The model under review builds one solid part; all positions refer to its coordinate system, in mm. Round coordinates to 2 decimals unless told otherwise and drop trailing zeros. Loops run counter-clockwise (first coordinate to the right, second up) from the corner with the lowest first, then second, coordinate; pieces in that order, holes last. Notation, with made-up numbers: M -31.75,67 L 5.25,67 A34 ccw 5.25,99 Z; hole C 52.25,64 d6. An arc over 180 degrees is marked long. Answer as a JSON object with one key per item and string values. Group by question number.
Item 1: Consider section B-B (x = 0). Give the boundary of the cut face in (y, z), and give its area (3 significant figures).
Item 2: Consider section D-D (x = 24). Give the boundary of the cut face in (y, z), and give its area (3 significant figures).
Item 3: Insertion check: P1, Ø1.8, axis at x = 33, z = -31, coming from the -Y side; P2, Ø1.6, axis at x = 38, y = 2, coming from the +Z side; P3, Ø0.9, axis at y = 2, z = -27, coming from the -X side; P4, Ø1.6, axis at x = -38.5, y = 2, coming from the -Z side. Each pin has a flat end and moves straight along its axis. Give the tip position at first contact, or say it passes through.
Item 4: Consider section C-C (z = 6.5). Give the boundary of the cut face in (x, y), and give its area (3 significant figures).
Item 5: Consider section A-A (z = 29). Give the boundary of the cut face in (x, y), and give its area (3 significant figures).
Item 6: To check wall thickness, follow line 1 (Z direction, x = 16.5, y = 1.85); line 2 (Z direction, x = 4, y = 1.3); line 3 (Z direction, x = -15.5, y = 0.75). State the ranges of each line that lie inside material, in increasing order.
```python
from build123d import *

# Parameters (mm, degrees)
SKETCH_2_R          = 11.05
SKETCH_2_R_2        = 2
SKETCH_2_R_3        = 4.5
SKETCH_2_R_4        = 1.5
EXTRUDE_1_DEPTH     = 3
SKETCH_3_R          = 1
CUT_EXTRUDE_1_DEPTH = 54.235326617
FILLET_1_R          = 1
FILLET_2_R          = 2


with BuildPart() as part:
    # 草图2 → 凸台-拉伸1 (new body)
    with BuildSketch(Plane(origin=(0, 0, 0), x_dir=(1, 0, 0), z_dir=(0, 1, 0))):
        Polygon((-37, 35), (37, 35), (37, 22.5), (40, 22.5), (40, 7.5), (37, 7.5), (37, -7.5), (40, -7.5), (40, -22.5), (37, -22.5), (37, -35), (-37, -35), (-37, -22.5), (-40, -22.5), (-40, -7.5), (-37, -7.5), (-37, 7.5), (-40, 7.5), (-40, 22.5), (-37, 22.5), align=None)
        with Locations(Location((0, 0, 0), (0, 0, 270))):
            Circle(SKETCH_2_R, mode=Mode.SUBTRACT)
        with Locations(Location((0, 29, 0), (0, 0, 270))):
            Circle(SKETCH_2_R_2, mode=Mode.SUBTRACT)
        with Locations(Location((0, 19.25, 0), (0, 0, 270))):
            Circle(SKETCH_2_R_3, mode=Mode.SUBTRACT)
        with Locations(Location((-33, 31, 0), (0, 0, 270))):
            Circle(SKETCH_2_R_4, mode=Mode.SUBTRACT)
        with Locations(Location((25.11473671, 14.5, 0), (0, 0, 270))):
            Circle(SKETCH_2_R_2, mode=Mode.SUBTRACT)
        with Locations(Location((16.670989023, 9.625, 0), (0, 0, 270))):
            Circle(SKETCH_2_R_3, mode=Mode.SUBTRACT)
        with Locations(Location((25.11473671, -14.5, 0), (0, 0, 270))):
            Circle(SKETCH_2_R_2, mode=Mode.SUBTRACT)
        with Locations(Location((16.670989023, -9.625, 0), (0, 0, 270))):
            Circle(SKETCH_2_R_3, mode=Mode.SUBTRACT)
        with Locations(Location((0, -29, 0), (0, 0, 270))):
            Circle(SKETCH_2_R_2, mode=Mode.SUBTRACT)
        with Locations(Location((0, -19.25, 0), (0, 0, 270))):
            Circle(SKETCH_2_R_3, mode=Mode.SUBTRACT)
        with Locations(Location((-25.11473671, -14.5, 0), (0, 0, 270))):
            Circle(SKETCH_2_R_2, mode=Mode.SUBTRACT)
        with Locations(Location((-16.670989023, -9.625, 0), (0, 0, 270))):
            Circle(SKETCH_2_R_3, mode=Mode.SUBTRACT)
        with Locations(Location((-25.11473671, 14.5, 0), (0, 0, 270))):
            Circle(SKETCH_2_R_2, mode=Mode.SUBTRACT)
        with Locations(Location((-16.670989023, 9.625, 0), (0, 0, 270))):
            Circle(SKETCH_2_R_3, mode=Mode.SUBTRACT)
        with Locations(Location((33, 31, 0), (0, 0, 90))):
            Circle(SKETCH_2_R_4, mode=Mode.SUBTRACT)
    extrude(amount=EXTRUDE_1_DEPTH)

    # 草图3 → 切除-拉伸1 (cut, through all)
    with BuildSketch(Plane(origin=(0, 3, 0), x_dir=(1, 0, 0), z_dir=(0, 1, 0))):
        with Locations((-37, 23.5)):
            Circle(SKETCH_3_R)
        with Locations((-37, 6.5)):
            Circle(SKETCH_3_R)
        with Locations((-37, -6.5)):
            Circle(SKETCH_3_R)
        with Locations((-37, -23.5)):
            Circle(SKETCH_3_R)
        with Locations((37, -23.5)):
            Circle(SKETCH_3_R)
        with Locations((37, -6.5)):
            Circle(SKETCH_3_R)
        with Locations((37, 6.5)):
            Circle(SKETCH_3_R)
        with Locations((37, 23.5)):
            Circle(SKETCH_3_R)
    extrude(amount=-CUT_EXTRUDE_1_DEPTH, mode=Mode.SUBTRACT)

    # 圆角1
    fillet_1_edges = [part.edges().sort_by_distance(p)[0] for p in [
        (40, 1.5, -22.5),
        (40, 1.5, -7.5),
        (40, 1.5, 7.5),
        (40, 1.5, 22.5),
        (-40, 1.5, 22.5),
        (-40, 1.5, 7.5),
        (-40, 1.5, -7.5),
        (-40, 1.5, -22.5),
    ]]
    fillet(fillet_1_edges, radius=FILLET_1_R)

    # 圆角2
    fillet_2_edges = [part.edges().sort_by_distance(p)[0] for p in [
        (-37, 1.5, -35),
        (37, 1.5, -35),
        (37, 1.5, 35),
        (-37, 1.5, 35),
    ]]
    fillet(fillet_2_edges, radius=FILLET_2_R)


solid = part.part
```
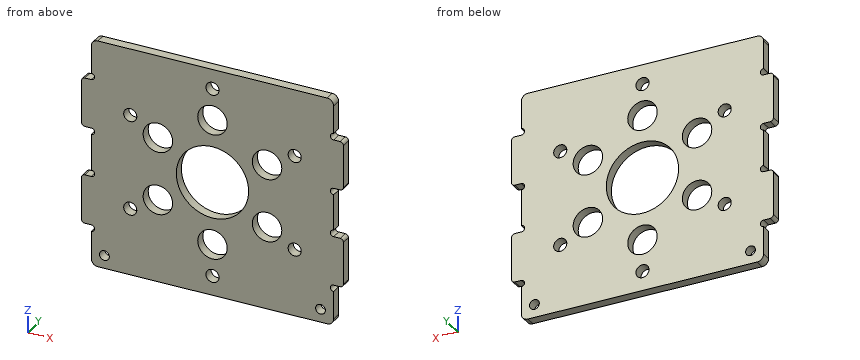
Geometry results:
{
 "1": {"outline": "M 0,-35 L 3,-35 L 3,-31 L 0,-31 Z; M 0,-27 L 3,-27 L 3,-23.75 L 0,-23.75 Z; M 0,-14.75 L 3,-14.75 L 3,-11.05 L 0,-11.05 Z; M 0,11.05 L 3,11.05 L 3,14.75 L 0,14.75 Z; M 0,23.75 L 3,23.75 L 3,27 L 0,27 Z; M 0,31 L 3,31 L 3,35 L 0,35 Z", "area": "65.7 mm^2"},
 "2": {"outline": "M 0,-35 L 3,-35 L 3,-16.16 L 0,-16.16 Z; M 0,-12.84 L 3,-12.84 L 3,12.84 L 0,12.84 Z; M 0,16.16 L 3,16.16 L 3,35 L 0,35 Z", "area": "190 mm^2"},
 "3": {"P1": "passes through", "P2": "stops at z = 22.5", "P3": "stops at x = -37", "P4": "stops at z = -22.5"},
 "4": {"outline": "M -36,0 L -19.91,0 L -19.91,3 L -36,3 Z; M -13.43,0 L -8.94,0 L -8.94,3 L -13.43,3 Z; M 8.94,0 L 13.43,0 L 13.43,3 L 8.94,3 Z; M 19.91,0 L 36,0 L 36,3 L 19.91,3 Z", "area": "124 mm^2"},
 "5": {"outline": "M -37,0 L -2,0 L -2,3 L -37,3 Z; M 2,0 L 37,0 L 37,3 L 2,3 Z", "area": "210 mm^2"},
 "6": {"line 1": "z = -35 to -14.12, -5.13 to 5.13, 14.12 to 35", "line 2": "z = -35 to -21.31, -17.19 to -10.3, 10.3 to 17.19, 21.31 to 35", "line 3": "z = -35 to -13.97, -5.28 to 5.28, 13.97 to 35"}
}
